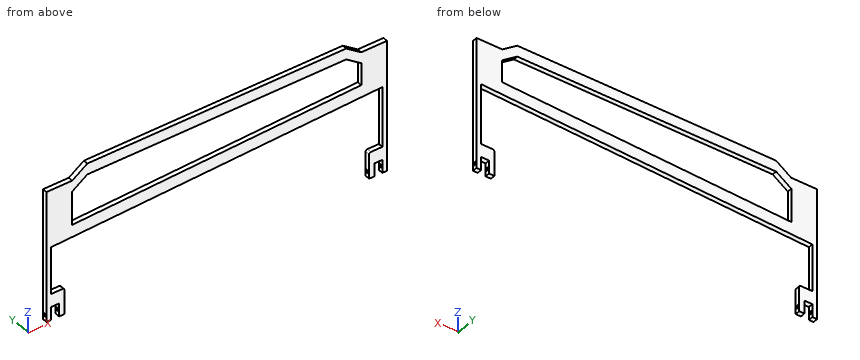
from build123d import *

# Parameters (mm, degrees)
F1_DEPTH = 9
F2_R     = 5.8193233161
F3_DEPTH = 1800


# Not quite as in the source:
# - a feature names something its author has since deleted; it is built from what else it names


with BuildPart() as f1:
    # F0 (on Front) → F1 (new body, symmetric)
    with BuildSketch(Plane.XZ):
        with BuildLine():
            Line((492.5543735346, 210), (0, 210))
            Line((0, 210), (-492.5543735346, 210))
            Line((-492.5543735346, 210), (-550, 170))
            Line((-550, 170), (-630, 170))
            Line((-630, 170), (-648, 170))
            Line((-648, 170), (-648, -230))
            Line((-648, -230), (-648, -330))
            Line((-648, -330), (-630, -330))
            Line((-630, -330), (-630, -280))
            Line((-630, -280), (-600, -280))
            Line((-600, -280), (-600, -330))
            Line((-600, -330), (-580, -330))
            Line((-580, -330), (-580, -236.35))
            ThreePointArc((-580, -236.35), (-581.8598719395, -231.8598719395), (-586.35, -230))
            Line((-586.35, -230), (-630, -230))
            Line((-630, -230), (-630, -50))
            Line((-630, -50), (630, 0))
            Line((630, 0), (630, -50))
            Line((630, -50), (630, -230))
            Line((630, -230), (586.35, -230))
            ThreePointArc((586.35, -230), (581.8598719395, -231.8598719395), (580, -236.35))
            Line((580, -236.35), (580, -330))
            Line((580, -330), (600, -330))
            Line((600, -330), (600, -280))
            Line((600, -280), (630, -280))
            Line((630, -280), (630, -330))
            Line((630, -330), (648, -330))
            Line((648, -330), (648, -230))
            Line((648, -230), (648, 170))
            Line((648, 170), (630, 170))
            Line((630, 170), (550, 170))
            Line((550, 170), (492.5543735346, 210))
        make_face()
        Polygon((550, 43.6507936508), (-550, 0), (-550, 128.1044334173), (-492.5543735346, 168.1044334173), (492.5543735346, 168.1044334173), (550, 128.1044334173), align=None, mode=Mode.SUBTRACT)
    extrude(amount=F1_DEPTH, both=True)

    # F2 (on face) → F3 (cut)
    with BuildSketch(Plane.YZ.offset(648)):
        with Locations((0, -307.489156723)):
            Circle(F2_R)
    extrude(amount=-F3_DEPTH, mode=Mode.SUBTRACT)


solid = f1.part
Can you work these out from the model? Positions are in its coordinate system, mm. Give positions to 0.01 mm unless a question says otherwise; leave off trailing zeros. Loops run counter-clockwise (first coordinate to the right, second up) from the corner with the lowest first, then second, coordinate; pieces in that order, holes last. Notation, with made-up numbers: (-35.75, -32.75) - (-11.75, -32.75) arc R32 cw to (-11.75, 5.25) - close; hole circle Ø9 at (-6.5, 54). An arc over 180 degrees is marked (long way). One line per item, written item: value.
(1) I'm going to push flat-ended pins straight in: pin 1 (3 mm diameter, centred on x = -497.5, y = -3.5, fed in from -Z); pin 2 (5.5 mm diameter, centred on x = -590, y = -2.5, fed in from +Z); pin 3 (5.5 mm diameter, centred on y = -1, z = -310, fed in from -X); pin 4 (9 mm diameter, centred on x = -208, y = 3, fed in from -Z). Where does each tip first touch, or does it pass through?
Verdict:
pin 1: z = -44.8
pin 2: z = 170
pin 3: through
pin 4: z = -33.43
(2) If we section it at A-A, the plane z = 17: List the corners of the cut face in (x, y) for me.
Verdict:
outline: (-648, -9) - (-550, -9) - (-550, 9) - (-648, 9) - close; (-121.6, -9) - (648, -9) - (648, 9) - (-121.6, 9) - close
(3) If we section it at B-B, the plane y = 0: State how many separate pieces and enclosed holes the cut face has, plus the area to 3 significant figures.
Verdict:
separate pieces: 5
enclosed holes: 1
area: 153,000 mm^2
(4) If we section it at C-C, the plane x = 121: List the corners of the cut face in (y, z) for me.
Verdict:
outline: (-9, -20.2) - (9, -20.2) - (9, 26.63) - (-9, 26.63) - close; (-9, 168.1) - (9, 168.1) - (9, 210) - (-9, 210) - close
(5) I need wall thicknesses on line 1 along X through (y, z) = (-1.75, -103.5); line 2 along Z through (x, y) = (-644, 0); line 3 along Z through (x, y) = (587.5, 0). Which ranges of each line are inside material? Lowest first, please.
Verdict:
line 1: -648 to -630, 630 to 648
line 2: -330 to -313.31, -301.67 to 170
line 3: -330 to -313.31, -301.67 to -230, -1.69 to 170
